Geometry: final body of the model. Coordinates: model frame, mm. Give positions to 0.01 mm unless a question says otherwise; leave off trailing zeros. Write each loop counter-clockwise with the first axis right and the second up, starting at its lowest first coordinate (ties: lowest second). Pieces come first, ordered by that corner, then holes.
Q1. Section C-C (x = -8.5). Return the cut outline in (y, z) (1 decimal).
Q2. Section D-D (z = 251). Return the cut outline in (x, y) (3 decimals).
Q3. Section B-B (y = 0.6). Return the cut outline in (x, z) (1 decimal).
Q4. Pin query (flat end, axial travel): pin 1 Ø1 at (x, y) = (-28, 1.5) entering from +Z. Return the tip coordinate at first contact, or that it passes through.
Q5. Line query: line 1 (X direction, y = 2.1, z = -264) (3 decimals); line 2 (X direction, y = 1.2, z = 252) (3 decimals); line 3 (Z direction, x = 20, y = 0.45). Output: solid intervals per line, ascending.
Q6. Section A-A (z = -240). Return the cut outline in (x, y) (3 decimals), plus the area to 3 significant figures.
from build123d import *

# Parameters (mm, degrees)
SKETCH1_W           = 758.19
SKETCH1_H           = 586.105
BOSS_EXTRUDE1_DEPTH = 3.175
CUT_EXTRUDE1_REACH  = 481.169
SKETCH2_W           = 127
SKETCH2_H           = 101.6
SKETCH2_W_2         = 127.178209898


with BuildPart() as part:
    # Sketch1 → Boss-Extrude1 (new body)
    with BuildSketch(Plane(origin=(0, 0, 0), x_dir=(1, 0, 0), z_dir=(0, 1, 0))):
        Rectangle(SKETCH1_W, SKETCH1_H)
    extrude(amount=BOSS_EXTRUDE1_DEPTH)

    # Sketch2 → Cut-Extrude1 (cut, up to next)
    with BuildSketch(Plane(origin=(0, 3.175, 0), x_dir=(1, 0, 0), z_dir=(0, 1, 0)), mode=Mode.PRIVATE) as cut_extrude1_sk1:
        with Locations((0, -242.2525)):
            Rectangle(SKETCH2_W, SKETCH2_H)
    cut_extrude1_tool1 = extrude(cut_extrude1_sk1.sketch, amount=-CUT_EXTRUDE1_REACH, mode=Mode.PRIVATE) & part.part
    # Sketch2 → Cut-Extrude1 (cut, up to next)
    with BuildSketch(Plane(origin=(0, 3.175, 0), x_dir=(1, 0, 0), z_dir=(0, 1, 0)), mode=Mode.PRIVATE) as cut_extrude1_sk2:
        with Locations((0.089104949, 242.2525)):
            Rectangle(SKETCH2_W_2, SKETCH2_H)
    cut_extrude1_tool2 = extrude(cut_extrude1_sk2.sketch, amount=-CUT_EXTRUDE1_REACH, mode=Mode.PRIVATE) & part.part
    add(cut_extrude1_tool1.solids().sort_by_distance((0, 3.175, 242.2525))[0], mode=Mode.SUBTRACT)
    add(cut_extrude1_tool2.solids().sort_by_distance((0.089105, 3.175, -242.2525))[0], mode=Mode.SUBTRACT)


solid = part.part
Computed:
1. outline: (0, -191.5) - (3.2, -191.5) - (3.2, 191.5) - (0, 191.5) - close
2. outline: (-379.095, 0) - (-63.5, 0) - (-63.5, 3.175) - (-379.095, 3.175) - close; (63.5, 0) - (379.095, 0) - (379.095, 3.175) - (63.5, 3.175) - close
3. outline: (-379.1, -293.1) - (-63.5, -293.1) - (-63.5, -191.5) - (63.7, -191.5) - (63.7, -293.1) - (379.1, -293.1) - (379.1, 293.1) - (63.5, 293.1) - (63.5, 191.5) - (-63.5, 191.5) - (-63.5, 293.1) - (-379.1, 293.1) - close
4. pin 1: stops at z = 191.45
5. line 1: x = -379.095 to -63.5, 63.678 to 379.095
5. line 2: x = -379.095 to -63.5, 63.5 to 379.095
5. line 3: z = -191.45 to 191.45
6. outline: (-379.095, 0) - (-63.5, 0) - (-63.5, 3.175) - (-379.095, 3.175) - close; (63.678, 0) - (379.095, 0) - (379.095, 3.175) - (63.678, 3.175) - close
6. area: 2,000 mm2
